The model under review builds one solid part; all positions refer to its coordinate system, in mm. Coordinates: 2 decimals unless noted, no trailing zeros. Loops run counter-clockwise (first coordinate to the right, second up) from the corner with the lowest first, then second, coordinate; pieces in that order, holes last. Notation, with made-up numbers: M 36.5,-11.75 L 89.5,-11.75 A14 cw 89.5,15.25 Z; hole C -21,48.5 d5. An arc over 180 degrees is marked long. One line per item, written item: value.
```python
from build123d import *

# Parameters (mm, degrees)
FILLET1_R = 1


with BuildPart() as part:
    # Sketch1 → Revolve1 (revolve)
    with BuildSketch(Plane.XY, mode=Mode.PRIVATE) as revolve1_sk:
        with BuildLine():
            Line((0, 13.938923092), (0, -14.5))
            ThreePointArc((0, -14.5), (14.275933158, -2.539238563), (5, 13.610657589))
            Line((5, 13.610657589), (5, 15.5))
            Line((5, 15.5), (14.275933158, 18.876163564))
            Line((14.275933158, 18.876163564), (14.275933158, 23.876163564))
            Line((14.275933158, 23.876163564), (11.775933158, 23.876163564))
            ThreePointArc((11.775933158, 23.876163564), (5.935541292, 22.752672467), (0, 22.376163564))
            Line((0, 22.376163564), (0, 13.938923092))
        make_face()
    revolve(revolve1_sk.sketch.rotate(Axis((0, 13.938923092, 0), (0, -1, 0)), 90), axis=Axis((0, 13.938923092, 0), (0, -1, 0)))

    # Fillet1
    fillet1_edges = [part.edges().sort_by_distance(p)[0] for p in [
        (0, 13.610657589, -5),
        (0, 23.876163564, -14.275933158),
        (0, 15.5, -5),
    ]]
    fillet(fillet1_edges, radius=FILLET1_R)


solid = part.part
```
(1) Insertion check: pin 1 Ø4 at (y, z) = (11.5, 1.5) entering from -X; pin 2 Ø8 at (y, z) = (-9, -1) entering from +X; pin 3 Ø4 at (x, y) = (8.5, 4.5) entering from -Z; pin 4 Ø1.5 at (x, y) = (9, 12.5) entering from +Z. Each pin has a flat end and moves straight along its axis. Give the tip position at first contact, or say it passes through.
Checks:
pin 1: x = -10.87
pin 2: x = 13.59
pin 3: z = -12.34
pin 4: through
(2) Add section A-A on y = -3. State the section outline as (x, z) points.
Checks:
outline: C 0,0 d28.37
(3) To check wall thickness, follow L1, parallel to Y at x = -2.25, z = 4.75; L2, parallel to Y at x = 10.5, z = -3; L3, parallel to X at y = 3.5, z = 6.25. State the ranges of each line that lie inside material, in increasing order. Write a range as [from, to].
Checks:
L1: [-13.51, 13.62], [15.47, 22.67]
L2: [-9.54, 9.54], [17.65, 23.66]
L3: [-12.61, 12.61]
(4) Draft analysis for pull direction Y (two halves, no side actions). For faces 1 (the face through (11, 23.876, -5)), 2 (the face through (-1.861, 15.936, 5.911)), 3 (the face through (-4.288, 20.904, 13.617)), state which applies: pulls with the +Y half, pulls with the -Y half, needs draft (parallel to the pull), parting line crosses it, or undercut.
Checks:
face 1: pulls with the +Y half
face 2: undercut
face 3: needs draft
(5) Add section B-B on y = 17.5. State the section outline as (x, z) points.
Checks:
outline: C 0,0 d20.99
